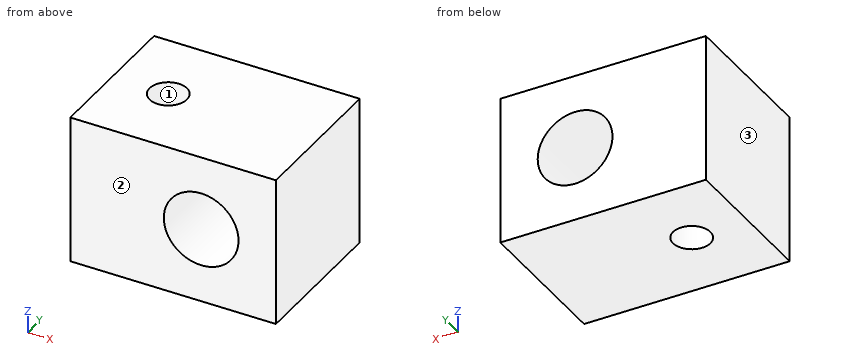
```python
from build123d import *

# Parameters (mm, degrees)
F0_R     = 6.35
F1_DEPTH = 25.4
F2_R     = 3.175
F3_DEPTH = 50.8


with BuildPart() as f1:
    # F0 (on Front) → F1 (new body)
    with BuildSketch(Plane.XZ):
        Polygon((28.463945, 9.493677), (-6.461055, 9.493677), (-6.461055, -15.906323), (28.463945, -15.906323), (28.463945, -3.206323), align=None)
        with Locations((15.763945, -3.206323)):
            Circle(F0_R, mode=Mode.SUBTRACT)
    extrude(amount=F1_DEPTH)

    # F2 (on face) → F3 (cut)
    with BuildSketch(Plane.XY.offset(9.493677)):
        with Locations((3.063945, -12.7)):
            Circle(F2_R)
    extrude(amount=-F3_DEPTH, mode=Mode.SUBTRACT)


solid = f1.part
```
Can you work these out from the model? Positions are in its coordinate system, mm. Face numbers are marked on the shaded views. Give positions to 0.01 mm unless a question says otherwise; leave off trailing zeros. Order: outer loops, then holes, each group sorted by start corner. A loop starts at its lowest first (then second) coordinate and runs counter-clockwise, first axis right, second up. Notation, with made-up numbers: M 5.5,33.25 L 44.5,33.25 A28 ccw 44.5,72.25 Z; hole C 14.25,53.5 d3. An arc over 180 degrees is marked long. Write item = value, one per line. Start each with the question number.
Q1. We'd pull the mould along X, two halves only. Please class the marked faces 1, 2 and 3: pulls with the +X half, pulls with the -X half, needs draft (parallel to the pull), parting line crosses it, or undercut.
Q2. Suppose I cut it at A-A (z = -1.75). Write out the boundary of the cut face in (x, y) (3 decimals).
Q3. Suppose I cut it at C-C (x = 4). Write out the boundary of the cut face in (y, z), plus the area to 3 significant figures.
Q4. I need wall thicknesses on probe 1 along Z at (x, y) = (17.5, -24); probe 2 along Z at (x, y) = (13, -24); probe 3 along Y at (x, z) = (5, -13.5). Which ranges of each line are inside material? Lowest first, please. Write a range as [from, to].
Q5. Suppose I cut it at B-B (y = -12.7). Write out the boundary of the cut face in (x, z).
Q6. Suppose I cut it at D-D (z = -11.25). Write out the boundary of the cut face in (x, y) (3 decimals), plus the area to 3 significant figures.
Check result:
q1.face_1 = undercut
q1.face_2 = needs draft
q1.face_3 = pulls with the -X half
q2.outline = M -6.461,-25.4 L 9.583,-25.4 L 9.583,0 L -6.461,0 Z; M 21.945,-25.4 L 28.464,-25.4 L 28.464,0 L 21.945,0 Z; hole C 3.064,-12.7 d6.35
q3.outline = M -25.4,-15.91 L -15.73,-15.91 L -15.73,9.49 L -25.4,9.49 Z; M -9.67,-15.91 L 0,-15.91 L 0,9.49 L -9.67,9.49 Z
q3.area = 491 mm2
q4.probe_1 = [-15.91, -9.31], [2.9, 9.49]
q4.probe_2 = [-15.91, -8.92], [2.51, 9.49]
q4.probe_3 = [-25.4, -15.22], [-10.18, 0]
q5.outline = M -6.46,-15.91 L -0.11,-15.91 L -0.11,9.49 L -6.46,9.49 Z; M 6.24,-15.91 L 28.46,-15.91 L 28.46,9.49 L 6.24,9.49 Z; hole C 15.76,-3.21 d12.7
q6.outline = M -6.461,-25.4 L 28.464,-25.4 L 28.464,0 L -6.461,0 Z; hole C 3.064,-12.7 d6.35
q6.area = 855 mm2
